```python
from build123d import *

# Parameters (mm, degrees)
SKETCH_1_R          = 8.4
EXTRUDE_1_DEPTH     = 18.5
EXTRUDE_START       = 1
SKETCH_2_R          = 2.5
EXTRUDE_2_DEPTH     = 1
EXTRUDE_4_DEPTH     = 3
SKETCH_3_R          = 1.5
CUT_EXTRUDE_1_DEPTH = 5
CUT_EXTRUDE_2_DEPTH = 2
CUT_EXTRUDE_3_DEPTH = 3


with BuildPart() as part:
    # Эскиз1 → Бобышка-Вытянуть1 (new, symmetric)
    with BuildSketch(Plane(origin=(0, 0, 0), x_dir=(0, 0, -1), z_dir=(1, 0, 0))):
        with BuildLine():
            Line((-8.95, -9.2), (8.95, -9.2))
            Line((8.95, -9.2), (12.95, -9.2))
            ThreePointArc((12.95, -9.2), (16.626955262, -7.676955262), (18.15, -4))
            Line((18.15, -4), (18.15, 0))
            ThreePointArc((18.15, 0), (15.455382387, 6.505382387), (8.95, 9.2))
            Line((8.95, 9.2), (-8.95, 9.2))
            ThreePointArc((-8.95, 9.2), (-15.455382387, 6.505382387), (-18.15, 0))
            Line((-18.15, 0), (-18.15, -4))
            ThreePointArc((-18.15, -4), (-16.626955262, -7.676955262), (-12.95, -9.2))
            Line((-12.95, -9.2), (-8.95, -9.2))
        make_face()
        with Locations((-8.95, 0)):
            Circle(SKETCH_1_R, mode=Mode.SUBTRACT)
        with Locations((8.95, 0)):
            Circle(SKETCH_1_R, mode=Mode.SUBTRACT)
        with BuildLine():
            Line((-1.93002849, -8.4), (1.93002849, -8.4))
            ThreePointArc((1.93002849, -8.4), (2.858869218, -7.770479287), (2.618260991, -6.674509804))
            ThreePointArc((2.618260991, -6.674509804), (1.659625246, -5.611633981), (0.87745098, -4.412930129))
            ThreePointArc((0.87745098, -4.412930129), (0, -3.892596448), (-0.87745098, -4.412930129))
            ThreePointArc((-0.87745098, -4.412930129), (-1.659625246, -5.611633981), (-2.618260991, -6.674509804))
            ThreePointArc((-2.618260991, -6.674509804), (-2.858869218, -7.770479287), (-1.93002849, -8.4))
        make_face(mode=Mode.SUBTRACT)
        with BuildLine():
            Line((-1.93002849, 8.4), (1.93002849, 8.4))
            ThreePointArc((1.93002849, 8.4), (2.858869218, 7.770479287), (2.618260991, 6.674509804))
            ThreePointArc((2.618260991, 6.674509804), (1.659625246, 5.611633981), (0.87745098, 4.412930129))
            ThreePointArc((0.87745098, 4.412930129), (0, 3.892596448), (-0.87745098, 4.412930129))
            ThreePointArc((-0.87745098, 4.412930129), (-1.659625246, 5.611633981), (-2.618260991, 6.674509804))
            ThreePointArc((-2.618260991, 6.674509804), (-2.858869218, 7.770479287), (-1.93002849, 8.4))
        make_face(mode=Mode.SUBTRACT)
    extrude(amount=EXTRUDE_1_DEPTH, both=True)

    # Эскиз2 → Бобышка-Вытянуть2 (add)
    with BuildSketch(Plane(origin=(18.5, 0, 0), x_dir=(0, 0, -1), z_dir=(1, 0, 0)).offset(EXTRUDE_START)):
        with BuildLine():
            Line((18.15, -4), (18.15, 0))
            ThreePointArc((18.15, 0), (15.455382387, 6.505382387), (8.95, 9.2))
            Line((8.95, 9.2), (-8.95, 9.2))
            ThreePointArc((-8.95, 9.2), (-15.455382387, 6.505382387), (-18.15, 0))
            Line((-18.15, 0), (-18.15, -4))
            ThreePointArc((-18.15, -4), (-16.626955262, -7.676955262), (-12.95, -9.2))
            Line((-12.95, -9.2), (12.95, -9.2))
            ThreePointArc((12.95, -9.2), (16.626955262, -7.676955262), (18.15, -4))
        make_face()
        with Locations((-8.95, 0)):
            Circle(SKETCH_2_R, mode=Mode.SUBTRACT)
        with Locations((8.95, 0)):
            Circle(SKETCH_2_R, mode=Mode.SUBTRACT)
    extrude(amount=-EXTRUDE_2_DEPTH)

    # Эскиз5 → Бобышка-Вытянуть4 (add, symmetric)
    with BuildSketch(Plane(origin=(-10, 0, 0), x_dir=(0, 0, -1), z_dir=(1, 0, 0))):
        with BuildLine():
            Line((-1.93002849, -8.4), (1.93002849, -8.4))
            ThreePointArc((1.93002849, -8.4), (2.858869218, -7.770479287), (2.618260991, -6.674509804))
            ThreePointArc((2.618260991, -6.674509804), (1.659625246, -5.611633981), (0.87745098, -4.412930129))
            ThreePointArc((0.87745098, -4.412930129), (0, -3.892596448), (-0.87745098, -4.412930129))
            ThreePointArc((-0.87745098, -4.412930129), (-1.659625246, -5.611633981), (-2.618260991, -6.674509804))
            ThreePointArc((-2.618260991, -6.674509804), (-2.858869218, -7.770479287), (-1.93002849, -8.4))
        make_face()
    extrude_4 = extrude(amount=EXTRUDE_4_DEPTH, both=True)

    # Зеркальное отражение1: Бобышка-Вытянуть4 across plane
    add(extrude_4.mirror(Plane(origin=(0, 0, 0), x_dir=(0, 0, 1), z_dir=(1, 0, 0))))

    # Эскиз3 → Вырез-Вытянуть1 (cut)
    with BuildSketch(Plane.XZ.offset(9.2)):
        with Locations(Location((-10, 0, 0), (0, 0, 270))):
            Circle(SKETCH_3_R)
        with Locations(Location((10, 0, 0), (0, 0, 90))):
            Circle(SKETCH_3_R)
    extrude(amount=-CUT_EXTRUDE_1_DEPTH, mode=Mode.SUBTRACT)

    # Эскиз6 → Вырез-Вытянуть2 (cut)
    with BuildSketch(Plane.ZY.offset(18.5)):
        with BuildLine():
            Line((11.45, -9.2), (6.45, -9.2))
            Line((6.45, -9.2), (6.45, -8.019351595))
            ThreePointArc((6.45, -8.019351595), (8.95, -8.4), (11.45, -8.019351595))
            Line((11.45, -8.019351595), (11.45, -9.2))
        make_face()
        with BuildLine():
            Line((-6.45, -8.019351595), (-6.45, -9.2))
            Line((-6.45, -9.2), (-11.45, -9.2))
            Line((-11.45, -9.2), (-11.45, -8.019351595))
            ThreePointArc((-11.45, -8.019351595), (-8.95, -8.4), (-6.45, -8.019351595))
        make_face()
    extrude(amount=-CUT_EXTRUDE_2_DEPTH, mode=Mode.SUBTRACT)

    # Эскиз7 → Вырез-Вытянуть3 (cut)
    with BuildSketch(Plane(origin=(19.5, 0, 0), x_dir=(0, 0, -1), z_dir=(1, 0, 0))):
        with BuildLine():
            Line((-6.45, -8.019351595), (-6.45, -9.2))
            Line((-6.45, -9.2), (-11.45, -9.2))
            Line((-11.45, -9.2), (-11.45, -8.019351595))
            ThreePointArc((-11.45, -8.019351595), (-8.95, -8.4), (-6.45, -8.019351595))
        make_face()
        with BuildLine():
            Line((11.45, -9.2), (6.45, -9.2))
            Line((6.45, -9.2), (6.45, -8.019351595))
            ThreePointArc((6.45, -8.019351595), (8.95, -8.4), (11.45, -8.019351595))
            Line((11.45, -8.019351595), (11.45, -9.2))
        make_face()
    extrude(amount=-CUT_EXTRUDE_3_DEPTH, mode=Mode.SUBTRACT)


solid = part.part
```
Can you work these out from the model? Positions are in its coordinate system, mm. A direction names the side the tool comes from. Coordinates: 2 decimals unless noted, no trailing zeros. Order: outer loops, then holes, each group sorted by start corner. A loop starts at its lowest first (then second) coordinate and runs counter-clockwise, first axis right, second up.
1. I need wall thicknesses on line 1 (Z direction, x = -9, y = 0); line 2 (Y direction, x = 19.05, z = -8.95); line 3 (Z direction, x = -11.5, y = 3.25). Which ranges of each line are inside material? Lowest first, please.
2. Thinking about a two-plate mould opening in X: for faces 6 (the face through (16, -8.4, 0)), 7 (the face through (18, -9, -11.45)), 8 (the face through (19.5, 0, 0)), which applies, +X half, -X half, draft (parallel to the pull), parting line (faces both ways), or undercut?
3. If we section it at B-B (z = -9.5): Please give me the cut outline in (x, y).
4. If we section it at A-A (x = -10): Please give me the cut outline in (y, z).
5. If we section it at D-D (x = 0): Please give me the cut outline in (y, z).
6. If we section it at C-C (y = 0.5): Please give me the cut outline in (x, z), then the cut area to 3 significant figures.
7. For faces 1 (the face through (1, -2, -18.15)), 2 (the face through (-11.464, -6.735, 0.325)), 3 (the face through (15.788, -3.893, -0.015)), 4 (the face through (-15.71, -7.79, -2.85)), 5 (the face through (1, 9.2, 0)), which set-ups out of +Z, -Z, +X, -X, +Y, -Y let a thin tool reach every point of the face, with its end or its side?
8. I'm going to push flat-ended pins straight in: pin 1 (1.5 mm diameter, centred on x = -10, z = 0.5, fed in from -Y); pin 2 (5 mm diameter, centred on y = 3, z = -12, fed in from -X); pin 3 (0.9 mm diameter, centred on x = 18.5, y = -8.5, fed in from -Z). Where does each tip first touch, or does it pass through?
Entries:
1. line 1: z = -18.15 to -17.35, -0.55 to 0.55, 17.35 to 18.15
1. line 2: y = -8.4 to -2.5, 2.5 to 9.2
1. line 3: z = -17.56 to -16.7, -1.2 to 1.2, 16.7 to 17.56
2. face 6: undercut
2. face 7: draft
2. face 8: +X half
3. outline: (-18.5, 8.38) - (18.5, 8.38) - (18.5, 2.44) - (19.5, 2.44) - (19.5, 9.18) - (-18.5, 9.18) - close; (-16.5, -9.2) - (16.5, -9.2) - (16.5, -8.38) - (-16.5, -8.38) - close; (18.5, -8.38) - (19.5, -8.38) - (19.5, -2.44) - (18.5, -2.44) - close
4. outline: (-9.2, -12.95) arc R5.2 ccw to (-4, -18.15) - (0, -18.15) arc R9.2 ccw to (9.2, -8.95) - (9.2, 8.95) arc R9.2 ccw to (0, 18.15) - (-4, 18.15) arc R5.2 ccw to (-9.2, 12.95) - (-9.2, 1.5) - (-4.2, 1.5) - (-4.2, -1.5) - (-9.2, -1.5) - close; hole circle Ø16.8 at (0, -8.95); hole circle Ø16.8 at (0, 8.95); hole (4.41, -0.88) arc R9.2 cw to (6.67, -2.62) arc R1 ccw to (8.4, -1.93) - (8.4, 1.93) arc R1 ccw to (6.67, 2.62) arc R9.2 cw to (4.41, 0.88) arc R1 ccw to start
5. outline: (-9.2, -12.95) arc R5.2 ccw to (-4, -18.15) - (0, -18.15) arc R9.2 ccw to (9.2, -8.95) - (9.2, 8.95) arc R9.2 ccw to (0, 18.15) - (-4, 18.15) arc R5.2 ccw to (-9.2, 12.95) - close; hole circle Ø16.8 at (0, -8.95); hole (-8.4, -1.93) arc R1 ccw to (-6.67, -2.62) arc R9.2 cw to (-4.41, -0.88) arc R1 ccw to (-4.41, 0.88) arc R9.2 cw to (-6.67, 2.62) arc R1 ccw to (-8.4, 1.93) - close; hole circle Ø16.8 at (0, 8.95); hole (4.41, -0.88) arc R9.2 cw to (6.67, -2.62) arc R1 ccw to (8.4, -1.93) - (8.4, 1.93) arc R1 ccw to (6.67, 2.62) arc R9.2 cw to (4.41, 0.88) arc R1 ccw to start
6. outline: (-18.5, -18.14) - (19.5, -18.14) - (19.5, -11.4) - (18.5, -11.4) - (18.5, -17.34) - (-18.5, -17.34) - close; (-18.5, -0.56) - (18.5, -0.56) - (18.5, -6.5) - (19.5, -6.5) - (19.5, 6.5) - (18.5, 6.5) - (18.5, 0.56) - (-18.5, 0.56) - close; (-18.5, 17.34) - (18.5, 17.34) - (18.5, 11.4) - (19.5, 11.4) - (19.5, 18.14) - (-18.5, 18.14) - close
6. area: 128 mm2
7. face 1: -Z, +X, -X, +Y, -Y
7. face 2: -Y
7. face 3: none
7. face 4: -X
7. face 5: +Z, -Z, +X, -X, +Y
8. pin 1: stops at y = -4.2
8. pin 2: stops at x = 18.5
8. pin 3: stops at z = -16.21
